The model under review builds one solid part; all positions refer to its coordinate system, in mm. Round coordinates to 2 decimals unless told otherwise and drop trailing zeros. Loops run counter-clockwise (first coordinate to the right, second up) from the corner with the lowest first, then second, coordinate; pieces in that order, holes last. Notation, with made-up numbers: (81.25, 36) -> (100.25, 36) arc R14 cw to (100.25, 62) -> close; hole circle Ø7 at (28.5, -8). An arc over 180 degrees is marked (long way). Use CSV: the item, a comma, the result in double quotes. Start each with the question number.
```python
from build123d import *

# Parameters (mm, degrees)
SKETCH1_W           = 160
SKETCH1_H           = 50
BOSS_EXTRUDE1_DEPTH = 1.25
SKETCH2_W           = 10
SKETCH2_H           = 2.5
SKETCH2_W_2         = 15
CUT_EXTRUDE1_DEPTH  = 4
SKETCH3_W           = 2.5
SKETCH3_H           = 22.5
CUT_EXTRUDE2_DEPTH  = 84.852549156
CUT_EXTRUDE3_REACH  = 85.853
SKETCH4_W           = 20
SKETCH4_H           = 11.5


with BuildPart() as part:
    # Sketch1 → Boss-Extrude1 (new, symmetric)
    with BuildSketch(Plane(origin=(0, 0, 0), x_dir=(1, 0, 0), z_dir=(0, 1, 0))):
        Rectangle(SKETCH1_W, SKETCH1_H)
    extrude(amount=BOSS_EXTRUDE1_DEPTH, both=True)

    # Sketch2 → Cut-Extrude1 (cut)
    with BuildSketch(Plane(origin=(0, 1.25, 0), x_dir=(1, 0, 0), z_dir=(0, 1, 0))):
        with Locations((30, 23.75)):
            Rectangle(SKETCH2_W, SKETCH2_H)
        with Locations((10, 23.75)):
            Rectangle(SKETCH2_W, SKETCH2_H)
        with Locations((10, -23.75)):
            Rectangle(SKETCH2_W, SKETCH2_H)
        with Locations((30, -23.75)):
            Rectangle(SKETCH2_W, SKETCH2_H)
        with Locations((50, 23.75)):
            Rectangle(SKETCH2_W, SKETCH2_H)
        with Locations((50, -23.75)):
            Rectangle(SKETCH2_W, SKETCH2_H)
        with Locations((-10, 23.75)):
            Rectangle(SKETCH2_W, SKETCH2_H)
        with Locations((-10, -23.75)):
            Rectangle(SKETCH2_W, SKETCH2_H)
        with Locations((-30, 23.75)):
            Rectangle(SKETCH2_W, SKETCH2_H)
        with Locations((-30, -23.75)):
            Rectangle(SKETCH2_W, SKETCH2_H)
        with Locations((-50, 23.75)):
            Rectangle(SKETCH2_W, SKETCH2_H)
        with Locations((-50, -23.75)):
            Rectangle(SKETCH2_W, SKETCH2_H)
        with Locations((72.5, 23.75)):
            Rectangle(SKETCH2_W_2, SKETCH2_H)
        with Locations((72.5, -23.75)):
            Rectangle(SKETCH2_W_2, SKETCH2_H)
        with Locations((-72.5, 23.75)):
            Rectangle(SKETCH2_W_2, SKETCH2_H)
        with Locations((-72.5, -23.75)):
            Rectangle(SKETCH2_W_2, SKETCH2_H)
    extrude(amount=-CUT_EXTRUDE1_DEPTH, mode=Mode.SUBTRACT)

    # Sketch3 → Cut-Extrude2 (cut, through all)
    with BuildSketch(Plane(origin=(0, 1.25, 0), x_dir=(1, 0, 0), z_dir=(0, 1, 0))):
        with Locations((78.75, -11.25)):
            Rectangle(SKETCH3_W, SKETCH3_H)
        with Locations((-78.75, -11.25)):
            Rectangle(SKETCH3_W, SKETCH3_H)
    extrude(amount=-CUT_EXTRUDE2_DEPTH, mode=Mode.SUBTRACT)

    # Sketch4 → Cut-Extrude3 (cut, up to next)
    with BuildSketch(Plane(origin=(0, -1.25, 0), x_dir=(-1, 0, 0), z_dir=(0, -1, 0)), mode=Mode.PRIVATE) as cut_extrude3_sk1:
        with Locations((37.5, 0)):
            Rectangle(SKETCH4_W, SKETCH4_H)
    cut_extrude3_tool1 = extrude(cut_extrude3_sk1.sketch, amount=-CUT_EXTRUDE3_REACH, mode=Mode.PRIVATE) & part.part
    add(cut_extrude3_tool1.solids().sort_by_distance((-37.5, -1.25, 0))[0], mode=Mode.SUBTRACT)


solid = part.part
```
1. For line 1 along X through (y, z) = (0.25, -2); line 2 along Z through (x, y) = (-33, 0.1); line 3 along X through (y, z) = (1.15, 2), list the stretches that pass through material, from the lowest coordinate up. Write a range as from..to.
2. Take a section at C-C, the plane z = 15. Give the boundary of the cut face in (x, y), then the cut area to 4 significant figures.
3. Take a section at B-B, the plane x = 10. Give the boundary of the cut face in (y, z), then the cut area to 4 significant figures.
4. Take a section at A-A, the plane z = 4. Give the boundary of the cut face in (x, y), then the cut area to 4 significant figures.
5. Clearance check with flat-ended pins moving along their axes: P1, Ø1, axis at y = -0.5, z = 9, coming from the -X side; P2, Ø1.2, axis at y = -0.5, z = -23.5, coming from the -X side; P3, Ø1.2, axis at x = -51.5, y = 0, coming from the -Z side; P4, Ø4, axis at x = -28.5, z = 5, coming from the -Y side. State where each tip first meets the part, or that it passes through.
Results:
1,line 1,"-80..-47.5, -27.5..80"
1,line 2,"-22.5..-5.75, 5.75..22.5"
1,line 3,"-77.5..-47.5, -27.5..77.5"
2,outline,"(-77.5, -1.25) -> (77.5, -1.25) -> (77.5, 1.25) -> (-77.5, 1.25) -> close"
2,area,"387.5 mm²"
3,outline,"(-1.25, -22.5) -> (1.25, -22.5) -> (1.25, 22.5) -> (-1.25, 22.5) -> close"
3,area,"112.5 mm²"
4,outline,"(-77.5, -1.25) -> (-47.5, -1.25) -> (-47.5, 1.25) -> (-77.5, 1.25) -> close; (-27.5, -1.25) -> (77.5, -1.25) -> (77.5, 1.25) -> (-27.5, 1.25) -> close"
4,area,"337.5 mm²"
5,P1,"x = -77.5"
5,P2,"x = -65"
5,P3,"z = -22.5"
5,P4,"y = -1.25"
